Input: part model. Units: mm. Frame: model coordinates. A direction names the side the tool comes from. Coordinates: 2 decimals unless noted, no trailing zeros. Order: outer loops, then holes, each group sorted by start corner. A loop starts at its lowest first (then second) coordinate and runs counter-clockwise, first axis right, second up. Notation, with made-up numbers: (73.5, -1.5) - (100.5, -1.5) arc R24 ccw to (100.5, 37.5) - close; hole circle Ø7 at (24, -5.5). An arc over 180 degrees is marked (long way). Use a Markdown table: item, result. Add a question column.
from build123d import *

# Parameters (mm, degrees)
SKETCH1_R                = 7
SKETCH1_R_2              = 5
BOSS_EXTRUDE1_DEPTH      = 8
CUT_EXTRUDE1_DEPTH       = 8
SKETCH5_W                = 9
SKETCH5_H                = 10
BOSS_EXTRUDE2_DEPTH      = 4
BOSS_EXTRUDE4_REACH      = 17.994
BOSS_EXTRUDE4_END_RADIUS = 7
SKETCH6_W                = 9
SKETCH6_H                = 4
SKETCH8_R                = 1
CUT_EXTRUDE2_DEPTH       = 8


with BuildPart() as part:
    # Sketch1 → Boss-Extrude1 (new body)
    with BuildSketch(Plane(origin=(0, 0, 0), x_dir=(1, 0, 0), z_dir=(0, 1, 0))):
        with Locations(Location((0, 0, 0), (0, 0, 270))):
            Circle(SKETCH1_R)
        with Locations(Location((0, 0, 0), (0, 0, 270))):
            Circle(SKETCH1_R_2, mode=Mode.SUBTRACT)
    extrude(amount=BOSS_EXTRUDE1_DEPTH)

    # Sketch2 → Cut-Extrude1 (cut)
    with BuildSketch(Plane(origin=(0, 8, 0), x_dir=(1, 0, 0), z_dir=(0, 1, 0))):
        Polygon((0, 0), (-4.949747468, 4.949747468), (-8.526445785, 8.526445785), (8.526445785, 8.526445785), align=None)
    extrude(amount=-CUT_EXTRUDE1_DEPTH, mode=Mode.SUBTRACT)



with BuildPart() as body_2:
    # Sketch5 → Boss-Extrude2 (new body)
    with BuildSketch(Plane(origin=(0, 0, 0), x_dir=(1, 0, 0), z_dir=(0, 1, 0))):
        with Locations((0.039670369, -12)):
            Rectangle(SKETCH5_W, SKETCH5_H)
    extrude(amount=BOSS_EXTRUDE2_DEPTH)


with BuildPart() as part_1:
    add(part.part)

    add(body_2.part)  # Boss-Extrude4 merges body 2
    # Boss-Extrude4: up to this cylinder (the profile starts outside it)
    boss_extrude4_end = Plane(origin=(0, 2, 0), z_dir=(0, -1, 0)) * Cylinder(BOSS_EXTRUDE4_END_RADIUS, 50.988, mode=Mode.PRIVATE)
    # Sketch6 → Boss-Extrude4 (add, up to the surface)
    with BuildSketch(Plane(origin=(0, 0, 7), x_dir=(-1, 0, 0), z_dir=(0, 0, -1)), mode=Mode.PRIVATE) as boss_extrude4_sk1:
        with Locations((-0.039670369, 2)):
            Rectangle(SKETCH6_W, SKETCH6_H)
    boss_extrude4_tool1 = extrude(boss_extrude4_sk1.sketch, amount=BOSS_EXTRUDE4_REACH, mode=Mode.PRIVATE) - boss_extrude4_end
    add(boss_extrude4_tool1.solids().sort_by_distance((0.03967, 2, 7))[0])
    add(boss_extrude4_tool1.solids().sort_by_distance((0.03967, 2, 7))[1])

    # Sketch8 → Cut-Extrude2 (cut)
    with BuildSketch(Plane(origin=(0, 4, 0), x_dir=(1, 0, 0), z_dir=(0, 1, 0))):
        with Locations(Location((0.048760734, -9.499904202, 0), (0, 0, 270))):
            Circle(SKETCH8_R)
        with Locations(Location((0.042700568, -14.499904202, 0), (0, 0, 270))):
            Circle(SKETCH8_R)
    extrude(amount=-CUT_EXTRUDE2_DEPTH, mode=Mode.SUBTRACT)


solid = part_1.part
1) Reachability of faces 4 (the flat face through (-4.46, 2, 11)), 5 (the cylindrical face through (0, 5, 7)), 6 (the flat face through (4.54, 2, 11)) from +Z, -Z, +X, -X, +Y, -Y: full face, straight path, thin tool, end or side. Return the list, or none.
2) Material intervals for L1, parallel to X at y = 5, z = 0; L2, parallel to Z at x = -0.25, y = 1.25; L3, parallel to X at y = 1.75, z = 9.5, sorted ascending.
3) Pull-direction query (Z, two-part tool) for faces 1 (the flat face through (-1, 0, 9)), 2 (the flat face through (-4, 4, -4)), 3 (the cylindrical face through (0.349, 2.028, 10.454)); classes: pulls with the +Z half, pulls with the -Z half, needs draft (parallel to the pull), parting line crosses it, or undercut.
4) Cut plane A-A (z = 0). Return the cut outline in (x, y).
5) Cut plane C-C (y = 3.5). Return the cut outline in (x, z).
6) Cut plane B-B (x = 4). Return the cut outline in (y, z).
7) Contact query for flat-ended pins moving along their axis: P1, Ø2, axis at y = 3, z = 10, coming from the +X side; P2, Ø1, axis at x = -2.5, z = 13.5, coming from the -Y side; P3, Ø2, axis at y = 1.5, z = 10.5, coming from the -X side; P4, Ø2, axis at y = 4, z = 2.5, coming from the +X side. Output: stop coordinate, or through.
8) Cut plane D-D (z = 6.5). Return the cut outline in (x, y).
Computed:
| question | item | result |
|---|---|---|
| 1 | face 4 | +Z, -X, +Y, -Y |
| 1 | face 5 | +Y |
| 1 | face 6 | +Z, +X, +Y, -Y |
| 2 | L1 | x = -7 to -5, 5 to 7 |
| 2 | L2 | z = 4.99 to 8.55, 10.45 to 13.54, 15.46 to 17 |
| 2 | L3 | x = -4.46 to -0.95, 1.05 to 4.54 |
| 3 | face 1 | needs draft |
| 3 | face 2 | pulls with the -Z half |
| 3 | face 3 | undercut |
| 4 | outline | (-7, 0) - (-5, 0) - (-5, 8) - (-7, 8) - close; (5, 0) - (7, 0) - (7, 8) - (5, 8) - close |
| 5 | outline | (-4.95, -4.95) - (-3.54, -3.54) arc R5 cw (long way) to (3.54, -3.54) - (4.95, -4.95) arc R7 ccw to (4.54, 5.33) - (4.54, 17) - (-4.46, 17) - (-4.46, 5.39) arc R7 ccw to start; hole circle Ø2 at (0.04, 14.5); hole circle Ø2 at (0.05, 9.5) |
| 6 | outline | (0, -4) - (8, -4) - (8, -3) - (0, -3) - close; (0, 3) - (8, 3) - (8, 5.74) - (4, 5.74) - (4, 17) - (0, 17) - close |
| 7 | P1 | stops at x = 4.54 |
| 7 | P2 | stops at y = 0 |
| 7 | P3 | stops at x = -4.46 |
| 7 | P4 | stops at x = 6.84 |
| 8 | outline | (-4.46, 0) - (4.54, 0) - (4.54, 4) - (2.6, 4) - (2.6, 8) - (-2.6, 8) - (-2.6, 4) - (-4.46, 4) - close |
